Here's the drawing with two shaded views (mm, measured from the low corner). I have some questions. Coordinates: 2 decimals unless noted, no trailing zeros. Write each loop counter-clockwise with the first axis right and the second up, starting at its lowest first coordinate (ties: lowest second). Pieces come first, ordered by that corner, then holes. Notation, with made-up numbers: M 30,-26 L 59,-26 A23 ccw 59,5 Z; hole C 63.25,54.5 d5. An arc over 180 degrees is marked long. Answer as CSV lines item,"result". Start each with the question number.
Item 1: Suppose I cut it at B-B, the plane y = 1.15. State how many separate pieces and enclosed holes the cut face has, and give its area (3 significant figures).
Item 2: Suppose I cut it at D-D, the plane z = 11. Write out the boundary of the cut face in (x, y).
Item 3: Suppose I cut it at A-A, the plane z = 32. Write out the boundary of the cut face in (x, y).
Item 4: Suppose I cut it at C-C, the plane x = 27. Write out the boundary of the cut face in (y, z).
Item 5: If I drill on line 1 along Z through (x, y) = (27, 0.8); line 2 along Z through (x, y) = (26.5, 0.75); line 3 along X through (y, z) = (0.35, 31.5), over which ranges is the centre line in solid material (lowest first)? Write a range as [from, to].
Item 6: I'm going to push a flat-ended pin straight in: P1, Ø1.8, axis at x = 27, z = 32, coming from the +Y side. Where does the tip first touch, or does it pass through?
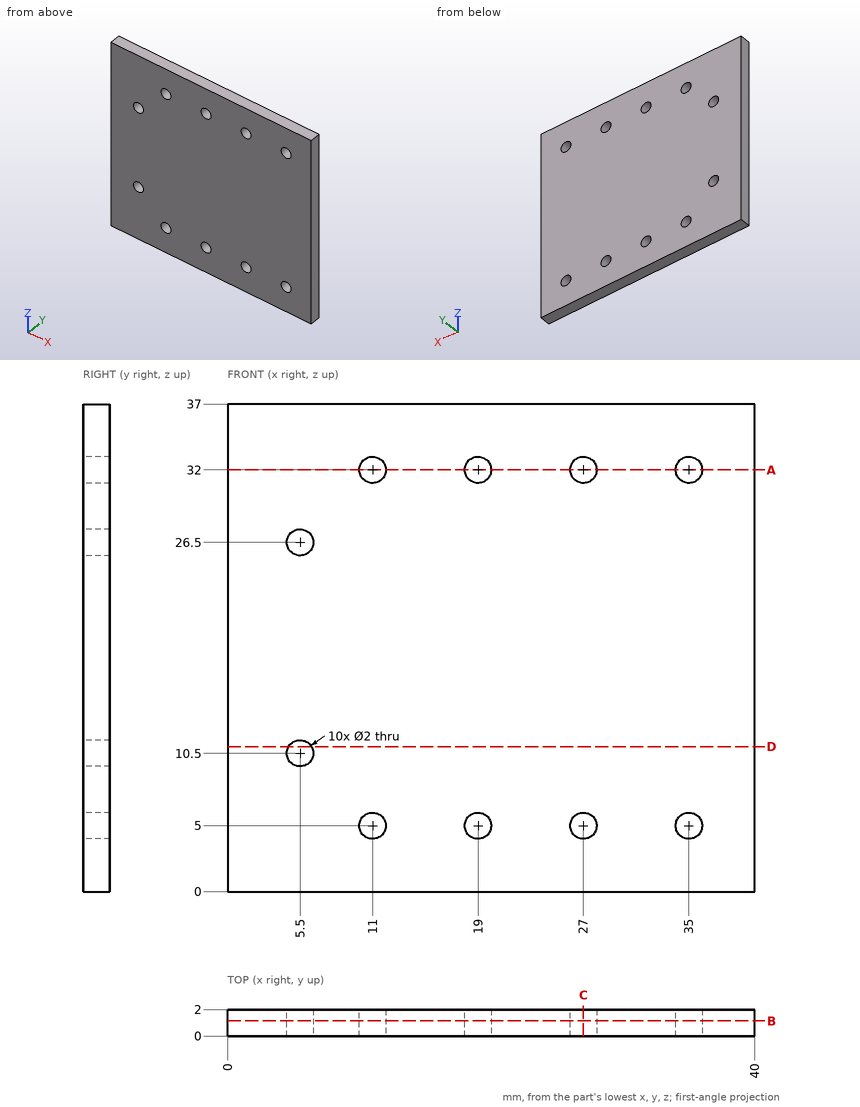
Ans:
1,separate pieces,"1"
1,enclosed holes,"10"
1,area,"1,450 mm^2"
2,outline,"M 0,0 L 4.63,0 L 4.63,2 L 0,2 Z; M 6.37,0 L 40,0 L 40,2 L 6.37,2 Z"
3,outline,"M 0,0 L 10,0 L 10,2 L 0,2 Z; M 12,0 L 18,0 L 18,2 L 12,2 Z; M 20,0 L 26,0 L 26,2 L 20,2 Z; M 28,0 L 34,0 L 34,2 L 28,2 Z; M 36,0 L 40,0 L 40,2 L 36,2 Z"
4,outline,"M 0,0 L 2,0 L 2,4 L 0,4 Z; M 0,6 L 2,6 L 2,31 L 0,31 Z; M 0,33 L 2,33 L 2,37 L 0,37 Z"
5,line 1,"z = [0, 4], [6, 31], [33, 37]"
5,line 2,"z = [0, 4.13], [5.87, 31.13], [32.87, 37]"
5,line 3,"x = [0, 10.13], [11.87, 18.13], [19.87, 26.13], [27.87, 34.13], [35.87, 40]"
6,P1,"passes through"
